from build123d import *

# Parameters (mm, degrees)
BOSS_EXTRUDE2_DEPTH              = 76.2
BOSS_EXTRUDE2_DEPTH_BACK         = 76.2
SKETCH6_W                        = 152.4
SKETCH6_H                        = 6.35
SKETCH6_W_2                      = 6.35
SKETCH6_H_2                      = 69.85
BOSS_EXTRUDE3_DEPTH              = 50.8
CUT_EXTRUDE3_REACH               = 84.55
CUT_EXTRUDE3_OFFSET_FROM_SURFACE = 6.35
SKETCH7_W                        = 127
SKETCH7_H                        = 69.85
BOSS_EXTRUDE5_DEPTH              = 57.15


with BuildPart() as part:
    # Sketch4 → Boss-Extrude2 (new body, two sides)
    with BuildSketch(Plane(origin=(0, 0, 0), x_dir=(0, 0, -1), z_dir=(1, 0, 0))) as boss_extrude2_sk:
        Polygon((0, 0), (0, 82.55), (-76.2, 82.55), align=None)
    extrude(amount=BOSS_EXTRUDE2_DEPTH)
    extrude(boss_extrude2_sk.sketch, amount=-BOSS_EXTRUDE2_DEPTH_BACK)

    # Sketch6 → Boss-Extrude3 (add)
    with BuildSketch(Plane(origin=(0, 0, 0), x_dir=(-1, 0, 0), z_dir=(0, 0, -1))):
        with Locations((0, 3.175)):
            Rectangle(SKETCH6_W, SKETCH6_H)
        with Locations((-66.675, 47.625)):
            Rectangle(SKETCH6_W_2, SKETCH6_H_2)
        with Locations((66.675, 47.625)):
            Rectangle(SKETCH6_W_2, SKETCH6_H_2)
    extrude(amount=BOSS_EXTRUDE3_DEPTH)

    # Cut-Extrude3: up to this face of the body (flat: up to its plane, moved by the offset)
    cut_extrude3_end = Plane(part.part.faces().sort_by_distance((0, 41.275, 38.1))[0]).offset(-CUT_EXTRUDE3_OFFSET_FROM_SURFACE)
    # Sketch7 → Cut-Extrude3 (cut, up to the picked face)
    with BuildSketch(Plane(origin=(0, 0, 0), x_dir=(-1, 0, 0), z_dir=(0, 0, -1)), mode=Mode.PRIVATE) as cut_extrude3_sk1:
        with Locations((0, 47.625)):
            Rectangle(SKETCH7_W, SKETCH7_H)
    cut_extrude3_tool1 = split(extrude(cut_extrude3_sk1.sketch, amount=-CUT_EXTRUDE3_REACH, mode=Mode.PRIVATE), bisect_by=cut_extrude3_end, keep=Keep.BOTH, mode=Mode.PRIVATE)
    add(cut_extrude3_tool1.solids().sort_by_distance((0, 47.625, 0))[0], mode=Mode.SUBTRACT)

    # Sketch8 → Boss-Extrude5 (add, symmetric)
    with BuildSketch(Plane(origin=(0, 41.275, 38.1), x_dir=(-1, 0, 0), z_dir=(0, -0.734803445, -0.678280103))):
        with BuildLine():
            Line((-53.798871559, 0), (-53.798871559, 25.4))
            Line((-53.798871559, 25.4), (53.798871559, 25.4))
            Line((53.798871559, 25.4), (53.798871559, 0))
            ThreePointArc((53.798871559, 0), (0, -53.798871559), (-53.798871559, 0))
        make_face()
    extrude(amount=BOSS_EXTRUDE5_DEPTH, both=True)


solid = part.part
The model under review builds one solid part; all positions refer to its coordinate system, in mm. A direction names the side the tool comes from. Coordinates: 2 decimals unless noted, no trailing zeros. Write each loop counter-clockwise with the first axis right and the second up, starting at its lowest first coordinate (ties: lowest second). Pieces come first, ordered by that corner, then holes. Notation, with made-up numbers: (-4.75, 83.5) - (27.25, 83.5) arc R24 ccw to (27.25, 100.5) - close; hole circle Ø9 at (78.25, 0). An arc over 180 degrees is marked (long way). Answer as a JSON object with one key per item and string values. Group by question number.
1. Add section A-A (z = -29.5). Give the boundary of the cut face in (x, y).
2. Clearance check with flat-ended pins moving along their axes: pin 1 Ø1.5 at (x, y) = (33.5, 24.5) entering from -Z; pin 2 Ø1 at (x, z) = (24, -33.5) entering from -Y; pin 3 Ø6.5 at (x, z) = (62, 19.5) entering from +Y. State where each tip first meets the part, or that it passes through.
3. To check wall thickness, follow probe 1 along X at (y, z) = (38.5, 23); probe 2 along X at (y, z) = (25, -2.5); probe 3 along X at (y, z) = (30, -35.5). State the ranges of each line that lie inside material, in increasing order.
4. Add section C-C (x = -20). Give the boundary of the cut face in (y, z), plus the area to 3 significant figures.
5. Mouldability with a two-part tool opening along Y and no side actions: class faces 5 (the face through (-0.8, 11.5, -13.9)), 6 (the face through (-0.75, -14.21, 13.95)), 7 (the face through (-69.85, 47, -25)) as pulls with the +Y half, pulls with the -Y half, needs draft (parallel to the pull), parting line crosses it, or undercut.
6. Add section B-B (x = -57). Give the boundary of the cut face in (y, z), plus the area to 3 significant figures.
7. Machinability: for faces 1 (the face through (-63.5, 55, -4)), 2 (the face through (-67, 82.55, 26)), 3 (the face through (67, 48, -50.8)), 4 (the face through (-67, 12.7, -25)), which of the approach directions +Z, -Z, +X, -X, +Y, -Y give a long, thin tool a straight path to every point of the face, cutting with its end or side? Answer none if there is none.
Findings:
{
 "1": {"outline": "(-76.2, 0) - (76.2, 0) - (76.2, 6.35) - (-76.2, 6.35) - close; (-69.85, 12.7) - (-63.5, 12.7) - (-63.5, 82.55) - (-69.85, 82.55) - close; (63.5, 12.7) - (69.85, 12.7) - (69.85, 82.55) - (63.5, 82.55) - close"},
 "2": {"pin 1": "z = -12.64", "pin 2": "y = 0", "pin 3": "y = 82.55"},
 "3": {"probe 1": "-76.2 to -63.5, -53.8 to 53.8, 63.5 to 76.2", "probe 2": "-69.85 to -63.5, -53.8 to 53.8, 63.5 to 69.85", "probe 3": "-69.85 to -63.5, 63.5 to 69.85"},
 "4": {"outline": "(-34.59, 36.03) - (0, -1.44) - (0, -50.8) - (6.35, -50.8) - (6.35, -8.32) - (16.51, -19.33) - (100.5, 58.2) - (49.39, 113.56) - close", "area": "8,900 mm²"},
 "5": {"face 5": "undercut", "face 6": "pulls with the -Y half", "face 7": "needs draft"},
 "6": {"outline": "(0, -50.8) - (6.35, -50.8) - (6.35, 0) - (12.7, 0) - (12.7, 3.08) - (82.55, 67.56) - (82.55, 76.2) - (0, 0) - close", "area": "1,000 mm²"},
 "7": {"face 1": "-Z, +Y", "face 2": "+Z, -Z, -X, +Y", "face 3": "-Z, +X, -X, +Y, -Y", "face 4": "-Z, -X"}
}
